Can you work these out from the model? Positions are in its coordinate system, mm. A direction names the side the tool comes from. Give positions to 0.01 mm unless a question says otherwise; leave off trailing zeros. Order: outer loops, then holes, each group sorted by start corner. A loop starts at its lowest first (then second) coordinate and runs counter-clockwise, first axis right, second up. Notation, with made-up numbers: M 88.5,82 L 121.5,82 A18 ccw 121.5,114 Z; hole C -33.5,64 d1. An arc over 180 degrees is marked long. Answer as a JSON object with one key per item and string values.
```python
from build123d import *

# Parameters (mm, degrees)
P_IDAT_VYSUNUT_M2_DEPTH  = 8
ZAOBLIT1_R               = 10
SKICA2_R                 = 1.65
SKICA2_R_2               = 10
ODEBRAT_VYSUNUT_M1_DEPTH = 8


with BuildPart() as part:
    # Skica1 → Přidat vysunutím2 (new body)
    with BuildSketch(Plane.XY):
        Polygon((0, 0), (210, 0), (210, 25), (180, 25), (180, 125), (210, 125), (210, 172), (180, 172), (180, 272), (210, 272), (210, 297), (0, 297), (0, 272), (30, 272), (30, 172), (0, 172), (0, 125), (30, 125), (30, 25), (0, 25), align=None)
    extrude(amount=P_IDAT_VYSUNUT_M2_DEPTH)

    # Zaoblit1
    zaoblit1_edges = [part.edges().sort_by_distance(p)[0] for p in [
        (0, 25, 4),
        (30, 25, 4),
        (30, 125, 4),
        (0, 125, 4),
        (0, 172, 4),
        (30, 172, 4),
        (30, 272, 4),
        (0, 272, 4),
        (0, 297, 4),
        (210, 297, 4),
        (210, 272, 4),
        (180, 272, 4),
        (180, 172, 4),
        (210, 172, 4),
        (210, 125, 4),
        (180, 125, 4),
        (180, 25, 4),
        (210, 25, 4),
        (210, 0, 4),
        (0, 0, 4),
    ]]
    fillet(zaoblit1_edges, radius=ZAOBLIT1_R)

    # Skica2 → Odebrat vysunutím1 (cut)
    with BuildSketch(Plane(origin=(0, 0, 0), x_dir=(-1, 0, 0), z_dir=(0, 0, -1))):
        with Locations((-173.6, 222)):
            Circle(SKICA2_R)
        with Locations((-36.4, 222)):
            Circle(SKICA2_R)
        with Locations((-55.45, 222)):
            Circle(SKICA2_R)
        with Locations((-154.55, 222)):
            Circle(SKICA2_R)
        with Locations((-173.6, 75)):
            Circle(SKICA2_R)
        with Locations((-154.55, 75)):
            Circle(SKICA2_R)
        with Locations((-55.45, 75)):
            Circle(SKICA2_R)
        with Locations((-36.4, 75)):
            Circle(SKICA2_R)
        with Locations((-105, 75)):
            Circle(SKICA2_R_2)
        with Locations((-105, 222)):
            Circle(SKICA2_R_2)
    extrude(amount=-ODEBRAT_VYSUNUT_M1_DEPTH, mode=Mode.SUBTRACT)


solid = part.part
```
1) I want a section at B-B on z = 3.5. Count the separate pieces of the cut face and the enclosed holes in it, and give its area (3 significant figures).
Results found:
{"separate pieces": "1", "enclosed holes": "10", "area": "49,600 mm²"}
2) For faces 1 (the face through (180, 74, 4)), 2 (the face through (112.37, 81.76, 3.94)), 3 (the face through (26.99, 122.15, 4.06)), which set-ups out of +Z, -Z, +X, -X, +Y, -Y let a thin tool reach every point of the face, with its end or its side?
Results found:
{"face 1": "+Z, -Z, +X", "face 2": "+Z, -Z", "face 3": "+Z, -Z, -X"}
3) I need wall thicknesses on L1, parallel to Y at x = 36.4, z = 1.5; L2, parallel to Y at x = 13, z = 5; L3, parallel to X at y = 215.5, z = 3.25. Which ranges of each line are inside material? Lowest first, please.
Results found:
{"L1": "y = 0 to 73.35, 76.65 to 220.35, 223.65 to 297", "L2": "y = 0 to 25, 125 to 172, 272 to 297", "L3": "x = 30 to 97.4, 112.6 to 180"}
4) Thinking about a two-plate mould opening in Y: for faces 4 (the face through (3.01, 2.85, 4.06)), 5 (the face through (104, 151, 0)), 6 (the face through (15, 172, 4)), which applies, pulls with the +Y half, pulls with the -Y half, needs draft (parallel to the pull), parting line crosses it, or undercut?
Results found:
{"face 4": "pulls with the -Y half", "face 5": "needs draft", "face 6": "undercut"}
5) I'm going to push flat-ended pins straight in: pin 1 Ø3 at (x, y) = (55.45, 75) entering from +Z; pin 2 Ø4 at (x, y) = (154.55, 75) entering from +Z; pin 3 Ø2.5 at (y, z) = (231.5, 6) entering from -X. Where does each tip first touch, or does it pass through?
Results found:
{"pin 1": "passes through", "pin 2": "stops at z = 8", "pin 3": "stops at x = 30"}
6) I want a section at A-A on y = 194.5. Write out the boundary of the cut face in (x, z).
Results found:
{"outline": "M 30,0 L 180,0 L 180,8 L 30,8 Z"}
